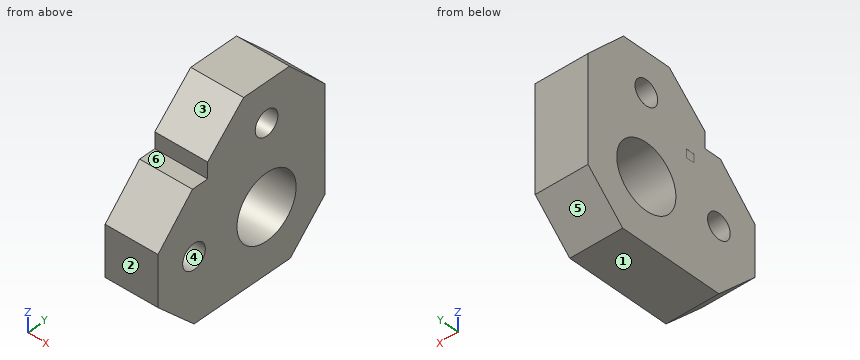
```python
from build123d import *

# Parameters (mm, degrees)
SKETCH1_R           = 3.9125
SKETCH1_R_2         = 1.5
BOSS_EXTRUDE1_DEPTH = 6.4
SKETCH2_W           = 1
SKETCH2_H           = 1
CUT_EXTRUDE1_DEPTH  = 0.01


with BuildPart() as part:
    # Sketch1 → Boss-Extrude1 (new body)
    with BuildSketch(Plane(origin=(0, 0, 0), x_dir=(0, 0, -1), z_dir=(1, 0, 0))):
        Polygon((9.255332298, -5.831457087), (4.574493559, -10.592295826), (-1.503828964, -10.592295826), (-6.264667702, -6.031457087), (-6.264667702, -4.026426966), (-8.199461444, -4.026426966), (-12.764667702, 0.738779293), (-12.764667702, 6.798306532), (-7.999461444, 11.483512791), (4.678092816, 11.483512791), (9.255332298, 6.898567055), align=None)
        with Locations((1.535332298, 3.768542913)):
            Circle(SKETCH1_R, mode=Mode.SUBTRACT)
        with Locations((-8.064667702, 3.768542913)):
            Circle(SKETCH1_R_2, mode=Mode.SUBTRACT)
        with Locations((1.535332298, -5.831457087)):
            Circle(SKETCH1_R_2, mode=Mode.SUBTRACT)
    extrude(amount=BOSS_EXTRUDE1_DEPTH)

    # Sketch2 → Cut-Extrude1 (cut)
    with BuildSketch(Plane.ZY):
        with Locations((4.264667702, -2.026426966)):
            Rectangle(SKETCH2_W, SKETCH2_H)
    extrude(amount=-CUT_EXTRUDE1_DEPTH, mode=Mode.SUBTRACT)


solid = part.part
```
Geometry: final body of the model. Coordinates: model frame, mm. Face numbers are marked on the shaded views. A direction names the side the tool comes from. Round coordinates to 2 decimals unless told otherwise and drop trailing zeros. Order: outer loops, then holes, each group sorted by start corner. A loop starts at its lowest first (then second) coordinate and runs counter-clockwise, first axis right, second up. Notation, with made-up numbers: M 59.25,2 L 77.25,2 A12 ccw 77.25,12 Z; hole C -11,44 d5. An arc over 180 degrees is marked long. Use one line per item in the form item = value. Start each with the question number.
Q1. Cut plane D-D (x = 2). Return loops of the section in (y, z) (1 decimal), and give its area (3 significant figures).
Q2. Cut plane C-C (y = 5). Return loops of the section in (x, z).
Q3. Pin query (flat end, axial travel): pin 1 Ø12.5 at (y, z) = (3.77, -1.54) entering from -X; pin 2 Ø1.8 at (y, z) = (-5.83, -1.54) entering from -X; pin 3 Ø1.5 at (x, z) = (5, 3.5) entering from -Y. Return the tip coordinate at first contact, or that it passes through.
Q4. Material intervals for line 1 (Z direction, x = 5.25, y = 4.75); line 2 (Y direction, x = 6.25, z = -2.5); line 3 (Y direction, x = 5, z = -4.25), sorted ascending. Write a range as [from, to].
Q5. Cut plane A-A (y = 1.5). Return loops of the section in (x, z), and give its area (3 significant figures).
Q6. Cut plane B-B (z = 2). Return loops of the section in (x, y), and give its area (3 significant figures).
Q7. Access query for the marked faces 5 and 6. Directions: +Z, -Z, +X, -X, +Y, -Y. A direction counts if a zero-diameter tool reaches every point of the face in a straight line with its end or side. Return the directions, or none.
Q8. Mould query, pull axis Z, two halves, no side actions, for the marked faces 1, 2, 3 and 4. Classes: +Z half, -Z half, draft (parallel to the pull), parting line (faces both ways), or undercut.
Geometry results:
q1.outline = M -10.6,-4.6 L -5.8,-9.3 L 6.9,-9.3 L 11.5,-4.7 L 11.5,8 L 6.8,12.8 L 0.7,12.8 L -4,8.2 L -4,6.3 L -6,6.3 L -10.6,1.5 Z; hole C -5.8,-1.5 d3; hole C 3.8,-1.5 d7.8; hole C 3.8,8.1 d3
q1.area = 327 mm^2
q2.outline = M 0,-9.26 L 6.4,-9.26 L 6.4,-5.25 L 0,-5.25 Z; M 0,2.18 L 6.4,2.18 L 6.4,7.21 L 0,7.21 Z; M 0,8.92 L 6.4,8.92 L 6.4,12.76 L 0,12.76 Z
q3.pin_1 = 0
q3.pin_2 = through
q3.pin_3 = -9.4
q4.line_1 = [-9.26, -5.32], [2.25, 6.93], [9.2, 12.76]
q4.line_2 = [-10.59, -6.98], [-4.68, -0.02], [7.56, 11.48]
q4.line_3 = [-10.59, 0.95], [6.59, 11.48]
q5.outline = M 0,-9.26 L 6.4,-9.26 L 6.4,-4.72 L 0,-4.72 Z; M 0,1.65 L 6.4,1.65 L 6.4,12.76 L 0,12.76 Z
q5.area = 100 mm^2
q6.outline = M 0,-10.12 L 6.4,-10.12 L 6.4,2.09 L 0,2.09 Z; M 0,5.44 L 6.4,5.44 L 6.4,11.48 L 0,11.48 Z
q6.area = 117 mm^2
q7.face_5 = -Z, +X, -X, +Y
q7.face_6 = +Z, +X, -X, -Y
q8.face_1 = -Z half
q8.face_2 = draft
q8.face_3 = +Z half
q8.face_4 = undercut
